from build123d import *

# Parameters (mm, degrees)
EXTRUDE_1_DEPTH   = 200
EXTRUDE_1_2_DEPTH = 18


with BuildPart() as part:
    # 草图1 → Extrude 1 (new body)
    with BuildSketch(Plane.XY):
        Polygon((78, 32), (83.5, 37.5), (83.5, 41.207106781), (72.707106781, 52), (0, 52), (-72.707106781, 52), (-83.5, 41.207106781), (-83.5, 37.5), (-78, 32), (-80.828427125, 29.171572875), (-87.5, 35.843145751), (-87.5, 42.863961031), (-74.363961031, 56), (0, 56), (74.363961031, 56), (87.5, 42.863961031), (87.5, 35.843145751), (80.828427125, 29.171572875), align=None)
    extrude(amount=-EXTRUDE_1_DEPTH)

    # 草图2 → Extrude 1 2 (add)
    with BuildSketch(Plane(origin=(0, 0, -200), x_dir=(-1, 0, 0), z_dir=(0, 0, -1))):
        Polygon((-8.414213562, 52), (3, 52), (3, 40.585786438), align=None)
    extrude(amount=-EXTRUDE_1_2_DEPTH)


solid = part.part
Here's how the part is built. I have some questions about the finished solid (model axes, mm). A direction names the side the tool comes from. Round coordinates to 2 decimals unless told otherwise and drop trailing zeros. Order: outer loops, then holes, each group sorted by start corner. A loop starts at its lowest first (then second) coordinate and runs counter-clockwise, first axis right, second up. Notation, with made-up numbers: (6.5, 27.25) -> (16.5, 27.25) arc R11 cw to (16.5, 38.25) -> close; hole circle Ø11 at (-18.5, 46.5). An arc over 180 degrees is marked (long way). Return JSON: item names as keys, results as strings.
Q1. If we section it at C-C on x = -0.5: List the corners of the cut face in (y, z) for me.
Filled sheet:
{"outline": "(43.09, -200) -> (56, -200) -> (56, 0) -> (52, 0) -> (52, -182) -> (43.09, -182) -> close"}
Q2. If we section it at A-A on y = 47.25: List the corners of the cut face in (x, z) for me.
Filled sheet:
{"outline": "(-83.11, -200) -> (-77.46, -200) -> (-77.46, 0) -> (-83.11, 0) -> close; (-3, -200) -> (3.66, -200) -> (3.66, -182) -> (-3, -182) -> close; (77.46, -200) -> (83.11, -200) -> (83.11, 0) -> (77.46, 0) -> close"}
Q3. I need wall thicknesses on line 1 along X through (y, z) = (39.5, -143.5); line 2 along Y through (x, z) = (59.5, -164); line 3 along X through (y, z) = (47, -156). Which ranges of each line are inside material? Lowest first, please. Write a range as from..to.
Filled sheet:
{"line 1": "x = -87.5..-83.5, 83.5..87.5", "line 2": "y = 52..56", "line 3": "x = -83.36..-77.71, 77.71..83.36"}
Q4. Which directions (+Z, -Z, +X, -X, +Y, -Y) give clear straight access to the entire face, cutting with the end or side of a thin tool? Please do faces 1 (the flat face through (81, 35, -99)), 2 (the flat face through (-3, 46, -191)), 3 (the flat face through (0, 50, -200)).
Filled sheet:
{"face 1": "+Z, -Z", "face 2": "+Z, -Z, -Y", "face 3": "-Z, +X, -X, +Y, -Y"}
Q5. For pin 1 Ø1 at (x, z) = (56, -90.5) entering from -Y; pin 2 Ø3.5 at (y, z) = (47, -189) entering from -X; pin 3 Ø5 at (y, z) = (45.5, -146.5) entering from -X, each with a flat end and sliding along its axis, tell me the tip position at first contact or that it passes through.
Filled sheet:
{"pin 1": "stops at y = 52", "pin 2": "stops at x = -85.11", "pin 3": "stops at x = -87.36"}
Q6. If we mould it in two halves opening along Y, with no side actions, what happens to faces 4 (the flat face through (-81.024, 49.34, -98.6)), 5 (the flat face through (-78.028, 46.679, -98.6)), 6 (the flat face through (1, 48, -182))? For each: released by +Y, released by -Y, zero draft, split by the parting line, or undercut.
Filled sheet:
{"face 4": "released by +Y", "face 5": "undercut", "face 6": "zero draft"}
Q7. If we section it at B-B on z = -81: List the corners of the cut face in (x, y) for me, plus the area to 3 significant figures.
Filled sheet:
{"outline": "(-87.5, 35.84) -> (-80.83, 29.17) -> (-78, 32) -> (-83.5, 37.5) -> (-83.5, 41.21) -> (-72.71, 52) -> (72.71, 52) -> (83.5, 41.21) -> (83.5, 37.5) -> (78, 32) -> (80.83, 29.17) -> (87.5, 35.84) -> (87.5, 42.86) -> (74.36, 56) -> (-74.36, 56) -> (-87.5, 42.86) -> close", "area": "835 mm^2"}
